For this review, take the finished solid that the model builds, in its own axes (mm). Face numbers are marked on the shaded views. A direction names the side the tool comes from. Round coordinates to 2 decimals unless told otherwise and drop trailing zeros. Write each loop counter-clockwise with the first axis right and the second up, starting at its lowest first coordinate (ties: lowest second). Pieces come first, ordered by that corner, then holes. Notation, with made-up numbers: M 78.5,79 L 86.5,79 A10 cw 86.5,91 Z; hole C 55,63 d2. An arc over 180 degrees is marked long. Answer in a Markdown table with one row per item.
Autodesk Inventor part; units mm, degrees
ref_plane "YZ Plane" through (0, 0, 0) normal (1, 0, 0) x (0, 1, 0)
ref_plane "XZ Plane" through (0, 0, 0) normal (0, 1, 0) x (-1, 0, 0)
ref_plane "XY Plane" through (0, 0, 0) normal (0, 0, 1) x (1, 0, 0)
sketch "Sketch1" plane through (0, 0, 0) normal (0, 0, 1) x (1, 0, 0)
  line L0 (-5, -11.1967) -> (-5, 0)
  arc A0 (-5, 0) -> (-6.8153, 3.8546) centre (-10, 0) ccw
  arc A1 (6.8153, 3.8546) -> (-6.8153, 3.8546) centre (0, 12.1033) ccw
  arc A2 (6.8153, 3.8546) -> (5, 0) centre (10, 0) ccw
  line L1 (5, 0) -> (5, -11.1967)
  line L2 (-2.5, -11.1967) -> (-2.5, 0)
  arc A3 (-2.5, 0) -> (-5.2229, 5.7818) centre (-10, 0) ccw
  arc A4 (5.2229, 5.7818) -> (-5.2229, 5.7818) centre (0, 12.1033) ccw
  arc A5 (5.2229, 5.7818) -> (2.5, 0) centre (10, 0) ccw
  line L3 (2.5, 0) -> (2.5, -11.1967)
  line L4 (-5, -11.1967) -> (-2.5, -11.1967)
  line L5 (2.5, -11.1967) -> (5, -11.1967)
  point P0 (0, 0)
  dimension "d2" = 10.7
  dimension "d4" = 10
  dimension "d5" = 5
  dimension "d7" = 2.5
  dimension "d16" = 34
extrude "Extrusion1" add sketch "Sketch1" along normal blind 48.5
sketch "Sketch2" plane through (-5, -11.1967, 0) normal (0, -1, 0) x (1, 0, 0)
  line L0 (2.5, 0) -> (0, 0)
  line L1 (2.5, 0) -> (2.5, 48.5)
  line L2 (0, 48.5) -> (2.5, 48.5)
  line L3 (0, 0) -> (0, 48.5)
  line L4 (10, 0) -> (7.5, 0)
  line L5 (10, 0) -> (10, 48.5)
  line L6 (7.5, 48.5) -> (10, 48.5)
  line L7 (7.5, 0) -> (7.5, 48.5)
  line L8 (-5.7, 0) -> (-5.7, 48.5)
  line L9 (15.7, 0) -> (15.7, 48.5)
  line L10 (-5.7, 48.5) -> (2.5, 48.5)
  line L11 (2.5, 48.5) -> (2.5, 30.5)
  line L12 (2.5, 30.5) -> (-5.7, 30.5)
  line L13 (-5.7, 30.5) -> (-5.7, 48.5)
  line L14 (7.5, 48.5) -> (15.7, 48.5)
  line L15 (15.7, 48.5) -> (15.7, 30.5)
  line L16 (15.7, 30.5) -> (7.5, 30.5)
  line L17 (7.5, 30.5) -> (7.5, 48.5)
  point P0 (5, 0)
  point P1 (-1.6, 30.5)
  dimension "d10" = 18
extrude "Extrusion2" cut sketch "Sketch2" against normal blind 48.5 contours L12 L3 L2 L1 | L12 L8 L10 L3 | L16 L7 L6 L5 | L5 L14 L9 L16
sketch "Sketch3" plane through (5, -11.1967, 0) normal (1, 0, 0) x (0, 0, -1)
  line L0 (0, 0) -> (0, 11.1967)
  line L1 (0, 11.1967) -> (-15.5, 0)
  line L2 (-15.5, 0) -> (0, 0)
  line L3 (0, 11.1967) -> (0, 0)
  line L4 (0, 0) -> (-30.5, 0)
  dimension "d18" = 15.5
extrude "Extrusion3" cut sketch "Sketch3" against normal blind 48.5
equation "\"BendRadius\" = Thickness"
equation "\"BendReliefWidth\" = Thickness"
equation "\"BendReliefDepth\" = 0.5 * Thickness"
equation "\"MinimumRemnant\" = 2 * Thickness"
equation "\"TransitionRadius\" = BendRadius"
equation "\"JacobiRadiusSize\" = BendRadius"
equation "\"GapSize\" = Thickness"
properties material "Iron, Gray"
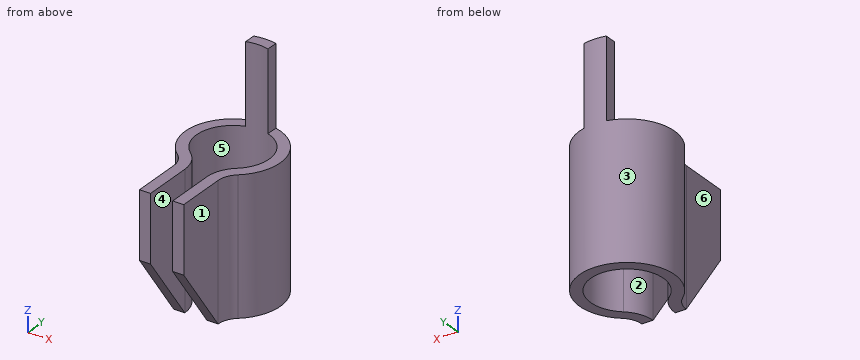
Q1. For probe 1 along Y at (x, z) = (0, 36.5); probe 2 along X at (y, z) = (-1, 21); probe 3 along Z at (x, y) = (8.5, 7), list the stretches that pass through material, from the lowest coordinate up.
Found:
| item | result |
|---|---|
| probe 1 | 20.3 to 22.8 |
| probe 2 | -5 to -2.5, 2.5 to 5 |
| probe 3 | 0 to 30.5 |
Q2. Machinability: for the marked faces 4, 5 and 6, which of the approach directions +Z, -Z, +X, -X, +Y, -Y give a long, thin tool a straight path to every point of the face, cutting with its end or side? Answer none if there is none.
Found:
| item | result |
|---|---|
| face 4 | +Z, -Z, -Y |
| face 5 | +Z, -Z |
| face 6 | +Z, -Z, -X, -Y |
Q3. Take a section at D-D (x = 0). State the section outline as (y, z) points, then the cut area to 3 significant figures.
Found:
| item | result |
|---|---|
| outline | M 20.3,0 L 22.8,0 L 22.8,48.5 L 20.3,48.5 Z |
| area | 121 mm² |
Q4. Take a section at C-C (z = 16.5). State the section outline as (x, y) points, then the cut area to 3 significant figures.
Found:
| item | result |
|---|---|
| outline | M -6.82,3.85 A5 cw -5,0 L -5,-11.2 L -2.5,-11.2 L -2.5,0 A7.5 ccw -5.22,5.78 A8.2 cw long 5.22,5.78 A7.5 ccw 2.5,0 L 2.5,-11.2 L 5,-11.2 L 5,0 A5 cw 6.82,3.85 A10.7 ccw long Z |
| area | 199 mm² |
Q5. Take a section at B-B (x = 5.75). State the section outline as (y, z) points, then the cut area to 3 significant figures.
Found:
| item | result |
|---|---|
| outline | M 2.63,0 L 6.26,0 L 6.26,30.5 L 2.63,30.5 Z; M 17.95,0 L 21.13,0 L 21.13,30.5 L 17.95,30.5 Z |
| area | 207 mm² |
Q6. Insertion check: P1, Ø6.5, axis at x = -8.5, y = 8.5, coming from the +Z side; P2, Ø3.5, axis at y = -5.5, z = 16, coming from the -X side; P3, Ø5, axis at x = -8, z = 17, coming from the +Y side. Each pin has a flat end and moves straight along its axis. Give the tip position at first contact, or say it passes through.
Found:
| item | result |
|---|---|
| P1 | z = 30.5 |
| P2 | x = -5 |
| P3 | y = 21.28 |
Q7. Take a section at A-A (y = -1.5). State the section outline as (x, z) points, then the cut area to 3 significant figures.
Found:
| item | result |
|---|---|
| outline | M -5,2.08 L -2.5,2.08 L -2.5,30.5 L -5,30.5 Z; M 2.5,2.08 L 5,2.08 L 5,30.5 L 2.5,30.5 Z |
| area | 142 mm² |
Q8. Mouldability with a two-part tool opening along X and no side actions: class the marked faces 1, 2 and 3 as +X half, -X half, draft (parallel to the pull), parting line (faces both ways), or undercut.
Found:
| item | result |
|---|---|
| face 1 | +X half |
| face 2 | undercut |
| face 3 | parting line |
